Geometry check sheet. Reference: drawing and pictorial views, mm from the part's lowest x, y, z. A direction names the side the tool comes from. Round coordinates to 2 decimals unless told otherwise and drop trailing zeros. Order: outer loops, then holes, each group sorted by start corner. A loop starts at its lowest first (then second) coordinate and runs counter-clockwise, first axis right, second up.
(1) Mould release check, pull along X, two halves, no side actions. Record for the marked faces 1, 2 and 3: released by +X, released by -X, zero draft, split by the parting line, or undercut.
(2) Sectioned sample at D-D, the plane x = 50.5. Enter the section's corners in (y, z).
(3) Sectioned sample at A-A, the plane z = 22.5. Enter the section's corners in (x, y), and give its area (3 significant figures).
(4) Thickness scan on probe 1 along Y at (x, z) = (21, 67.5); probe 2 along X at (y, z) = (64, 72); probe 3 along Z at (x, y) = (29, 61.5). Record the ranges inside material, lowest first.
(5) Depth check by flat-ended pin: pin 1 (10 mm diameter, centred on y = 66, z = 17.5, fed in from -X); pin 2 (10 mm diameter, centred on x = 29, y = 91.5, fed in from +Z). Enter the tip coordinate at first touch or a pass-through.
(6) Tool access check on the marked faces 4 and 5. Record the directions out of +Z, -Z, +X, -X, +Y, -Y that give a thin tool (end or side, any length) a straight path to the whole face; none if there is none.
(7) Sectioned sample at B-B, the plane y = 52. Enter the section's corners in (x, z).
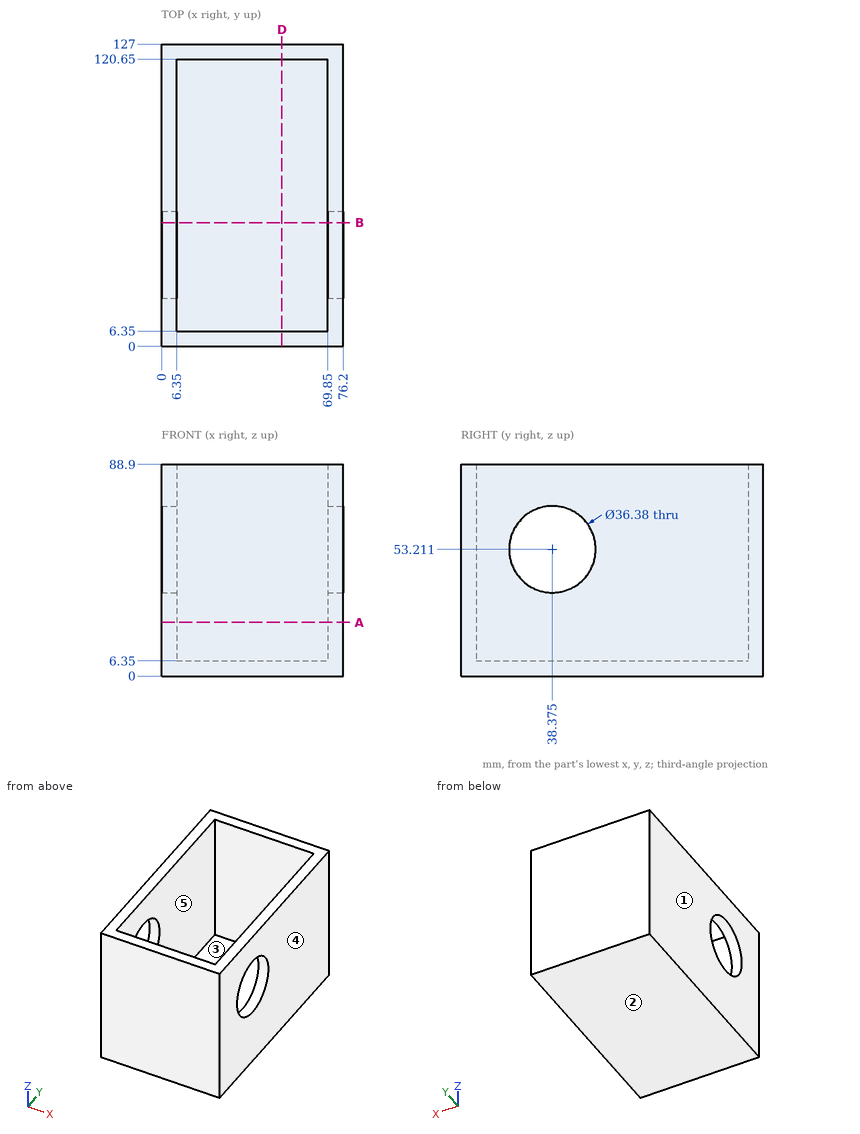
Derived:
1. face 1: released by -X
1. face 2: zero draft
1. face 3: undercut
2. outline: (0, 0) - (127, 0) - (127, 88.9) - (120.65, 88.9) - (120.65, 6.35) - (6.35, 6.35) - (6.35, 88.9) - (0, 88.9) - close
3. outline: (0, 0) - (76.2, 0) - (76.2, 127) - (0, 127) - close; hole (6.35, 6.35) - (69.85, 6.35) - (69.85, 120.65) - (6.35, 120.65) - close
3. area: 2,420 mm2
4. probe 1: y = 0 to 6.35, 120.65 to 127
4. probe 2: x = 0 to 6.35, 69.85 to 76.2
4. probe 3: z = 0 to 6.35
5. pin 1: stops at x = 0
5. pin 2: stops at z = 6.35
6. face 4: +Z, -Z, +X, +Y, -Y
6. face 5: +Z
7. outline: (0, 0) - (76.2, 0) - (76.2, 41.16) - (69.85, 41.16) - (69.85, 6.35) - (6.35, 6.35) - (6.35, 41.16) - (0, 41.16) - close; (0, 65.26) - (6.35, 65.26) - (6.35, 88.9) - (0, 88.9) - close; (69.85, 65.26) - (76.2, 65.26) - (76.2, 88.9) - (69.85, 88.9) - close
